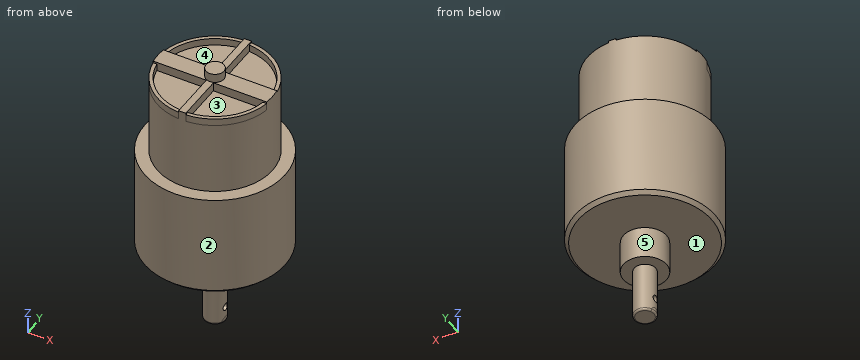
from build123d import *
from build123d.topology import SkipClean

# Parameters (mm, degrees)
SKETCH1_R               = 16
BOSS_EXTRUDE1_DEPTH     = 23
SKETCH2_R               = 19.5
BOSS_EXTRUDE2_DEPTH     = 29
SKETCH3_R               = 6
BOSS_EXTRUDE4_DEPTH     = 9
SKETCH4_R               = 3
BOSS_EXTRUDE5_DEPTH     = 22
CUT_EXTRUDE2_DEPTH      = 22
CUT_EXTRUDE2_DEPTH_BACK = 22
SKETCH5_R               = 1.5
CUT_EXTRUDE4_START      = -2.5
CUT_EXTRUDE4_DEPTH      = 2.5
SKETCH7_R               = 2.5
BOSS_EXTRUDE6_DEPTH     = 2.5
BOSS_EXTRUDE7_DEPTH     = 2
CHAMFER1_SIZE           = 1
FILLET1_R               = 1
BOSS_EXTRUDE8_START     = -22
SKETCH9_R               = 3
BOSS_EXTRUDE8_DEPTH     = 22
CUT_EXTRUDE6_START      = -8
SKETCH10_R              = 3
CUT_EXTRUDE6_DEPTH      = 8
FILLET2_R               = 0.5
CUT_EXTRUDE7_DEPTH      = 59.860003398
CUT_EXTRUDE7_DEPTH_BACK = 59.860003398
SKETCH11_R              = 1


with BuildPart() as part:
    # Sketch1 → Boss-Extrude1 (new body)
    with BuildSketch(Plane.XY):
        Circle(SKETCH1_R)
    extrude(amount=BOSS_EXTRUDE1_DEPTH)

    # Sketch2 → Boss-Extrude2 (add)
    with BuildSketch(Plane(origin=(0, 0, 0), x_dir=(-1, 0, 0), z_dir=(0, 0, -1))):
        with Locations(Location((0, 0, 0), (0, 0, 180))):
            Circle(SKETCH2_R)
    extrude(amount=BOSS_EXTRUDE2_DEPTH)

    # Sketch3 → Boss-Extrude4 (add)
    with BuildSketch(Plane(origin=(0, 0, -29), x_dir=(-1, 0, 0), z_dir=(0, 0, -1))):
        Circle(SKETCH3_R)
    extrude(amount=BOSS_EXTRUDE4_DEPTH)

    # Sketch4 → Boss-Extrude5 (add)
    with BuildSketch(Plane(origin=(0, 0, -38), x_dir=(-1, 0, 0), z_dir=(0, 0, -1))):
        Circle(SKETCH4_R)
    extrude(amount=BOSS_EXTRUDE5_DEPTH)

    # Sketch5 → Cut-Extrude2 (cut, two sides: drawn at the far end of the back side and taken through both)
    with BuildSketch(Plane(origin=(0, 0, 0), x_dir=(0, 0, -1), z_dir=(1, 0, 0)).offset(-CUT_EXTRUDE2_DEPTH_BACK)):
        with Locations((52, 0)):
            Circle(SKETCH5_R)
    extrude(amount=CUT_EXTRUDE2_DEPTH + CUT_EXTRUDE2_DEPTH_BACK, mode=Mode.SUBTRACT)

    # Sketch6 → Cut-Extrude4 (cut)
    with BuildSketch(Plane.XY.offset(23).offset(CUT_EXTRUDE4_START)):
        with BuildLine():
            Line((0.998052578, -2.481549033), (0.998052578, -15.968841256))
            ThreePointArc((0.998052578, -15.968841256), (10.773767775, -11.829029036), (15.806388405, -2.481549033))
            Line((15.806388405, -2.481549033), (0.998052578, -2.481549033))
        make_face()
        with BuildLine():
            Line((-0.998052578, 15.968841256), (-0.998052578, 2.481549033))
            Line((-0.998052578, 2.481549033), (-15.806388405, 2.481549033))
            ThreePointArc((-15.806388405, 2.481549033), (-10.773767775, 11.829029036), (-0.998052578, 15.968841256))
        make_face()
        with BuildLine():
            Line((0.998052578, 15.968841256), (0.998052578, 2.481549033))
            Line((0.998052578, 2.481549033), (15.806388405, 2.481549033))
            ThreePointArc((15.806388405, 2.481549033), (10.773767775, 11.829029036), (0.998052578, 15.968841256))
        make_face()
        with BuildLine():
            Line((-15.806388405, -2.481549033), (-0.998052578, -2.481549033))
            Line((-0.998052578, -2.481549033), (-0.998052578, -15.968841256))
            ThreePointArc((-0.998052578, -15.968841256), (-10.773767775, -11.829029036), (-15.806388405, -2.481549033))
        make_face()
    extrude(amount=CUT_EXTRUDE4_DEPTH, mode=Mode.SUBTRACT)

    # Sketch7 → Boss-Extrude6 (add)
    with BuildSketch(Plane.XY.offset(23)):
        Circle(SKETCH7_R)
    extrude(amount=BOSS_EXTRUDE6_DEPTH)

    # Sketch8 → Boss-Extrude7 (add)
    with BuildSketch(Plane.XY.offset(20.5)):
        with BuildLine():
            Line((-15.806388405, 2.481549033), (-14.793306405, 2.481549033))
            ThreePointArc((-14.793306405, 2.481549033), (-10.065380021, 11.12151631), (-0.998052578, 14.966759537))
            Line((-0.998052578, 14.966759537), (-0.998052578, 15.968841256))
            ThreePointArc((-0.998052578, 15.968841256), (-10.773767775, 11.829029036), (-15.806388405, 2.481549033))
        make_face()
        with BuildLine():
            Line((0.998052578, 15.968841256), (0.998052578, 14.966759537))
            ThreePointArc((0.998052578, 14.966759537), (10.065380021, 11.12151631), (14.793306405, 2.481549033))
            Line((14.793306405, 2.481549033), (15.806388405, 2.481549033))
            ThreePointArc((15.806388405, 2.481549033), (10.773767775, 11.829029036), (0.998052578, 15.968841256))
        make_face()
        with BuildLine():
            Line((15.806388405, -2.481549033), (14.793306405, -2.481549033))
            ThreePointArc((14.793306405, -2.481549033), (10.065380021, -11.12151631), (0.998052578, -14.966759537))
            Line((0.998052578, -14.966759537), (0.998052578, -15.968841256))
            ThreePointArc((0.998052578, -15.968841256), (10.773767775, -11.829029036), (15.806388405, -2.481549033))
        make_face()
        with BuildLine():
            Line((-0.998052578, -15.968841256), (-0.998052578, -14.966759537))
            ThreePointArc((-0.998052578, -14.966759537), (-10.065380021, -11.12151631), (-14.793306405, -2.481549033))
            Line((-14.793306405, -2.481549033), (-15.806388405, -2.481549033))
            ThreePointArc((-15.806388405, -2.481549033), (-10.773767775, -11.829029036), (-0.998052578, -15.968841256))
        make_face()
    extrude(amount=BOSS_EXTRUDE7_DEPTH)

    # Chamfer1
    chamfer1_edges = [part.edges().sort_by_distance(p)[0] for p in [
        (-19.5, 0, -29),
    ]]
    chamfer(chamfer1_edges, length=CHAMFER1_SIZE)

    # Fillet1
    fillet1_edges = [part.edges().sort_by_distance(p)[0] for p in [
        (3, 0, -60),
    ]]
    fillet(fillet1_edges, radius=FILLET1_R)

    # Sketch9 → Boss-Extrude8 (add)
    with SkipClean():  # the faces are left unmerged after this step: merging them gives an invalid solid
        with BuildSketch(Plane(origin=(0, 0, -60), x_dir=(-1, 0, 0), z_dir=(0, 0, -1)).offset(BOSS_EXTRUDE8_START)):
            Circle(SKETCH9_R)
        extrude(amount=BOSS_EXTRUDE8_DEPTH)

    # Sketch10 → Cut-Extrude6 (cut)
    with BuildSketch(Plane(origin=(0, 0, -60), x_dir=(-1, 0, 0), z_dir=(0, 0, -1)).offset(CUT_EXTRUDE6_START)):
        Circle(SKETCH10_R)
    extrude(amount=CUT_EXTRUDE6_DEPTH, mode=Mode.SUBTRACT)

    # Fillet2
    fillet2_edges = [part.edges().sort_by_distance(p)[0] for p in [
        (3, 0, -52),
    ]]
    fillet(fillet2_edges, radius=FILLET2_R)

    # Sketch11 → Cut-Extrude7 (cut, two sides: drawn at the far end of the back side and taken through both)
    with BuildSketch(Plane(origin=(0, 0, 0), x_dir=(0, 0, -1), z_dir=(1, 0, 0)).offset(-CUT_EXTRUDE7_DEPTH_BACK)):
        with Locations((47.584115537, 0)):
            Circle(SKETCH11_R)
    extrude(amount=CUT_EXTRUDE7_DEPTH + CUT_EXTRUDE7_DEPTH_BACK, mode=Mode.SUBTRACT)


solid = part.part
Geometry check sheet. Reference: the model listing, model coordinates, mm. Face numbers are marked on the shaded views. A direction names the side the tool comes from. Give positions to 0.01 mm unless a question says otherwise; leave off trailing zeros. Loops run counter-clockwise (first coordinate to the right, second up) from the corner with the lowest first, then second, coordinate; pieces in that order, holes last. Notation, with made-up numbers: M -22,19.5 L 21,19.5 A20 cw 21,39.5 Z; hole C 59,51.25 d8. An arc over 180 degrees is marked long. Answer as a JSON object with one key per item and string values. Group by question number.
Item 1: Access from +Z, -Z, +X, -X, +Y, -Y to the whole of each face (thin tool, end or side, straight path). Record for the marked faces 4 and 5.
Item 2: Material ranges on L1, parallel to Y at x = -2.5, z = 21.5; L2, parallel to Z at x = 0.75, y = 0; L3, parallel to Y at x = -9, z = 22, recorded low to high.
Item 3: Sectioned sample at A-A on y = 0. Record the boundary of the cut face in (x, z).
Item 4: Sectioned sample at B-B on x = 0. Record the boundary of the cut face in (y, z).
Item 5: Sectioned sample at C-C on z = -19. Record the boundary of the cut face in (x, y).
Item 6: Gauge pin test, flat ends, axial feed: pin 1 (1.5 mm diameter, centred on x = -5.5, y = 6.5, fed in from +Z); pin 2 (1.2 mm diameter, centred on x = -5, z = 22, fed in from +Y); pin 3 (4 mm diameter, centred on y = -10.5, z = -31.5, fed in from -X); pin 4 (6 mm diameter, centred on y = 6, z = -2, fed in from +X). Record the tip position at first contact, or that the pin passes through.
Item 7: Mould release check, pull along X, two halves, no side actions. Record for the marked faces 1, 2 and 3: pulls with the +X half, pulls with the -X half, needs draft (parallel to the pull), parting line crosses it, or undercut.
Findings below:
{
 "1": {"face 4": "+Z", "face 5": "-Z"},
 "2": {"L1": "-15.8 to -14.79, -2.48 to 2.48, 14.79 to 15.8", "L2": "-52 to -48.58, -46.58 to 25.5", "L3": "-13.23 to -12, -2.48 to 2.48, 12 to 13.23"},
 "3": {"outline": "M -19.5,-28 L -18.5,-29 L -6,-29 L -6,-38 L -3,-38 L -3,-46.58 L 3,-46.58 L 3,-38 L 6,-38 L 6,-29 L 18.5,-29 L 19.5,-28 L 19.5,0 L 16,0 L 16,23 L 2.5,23 L 2.5,25.5 L -2.5,25.5 L -2.5,23 L -16,23 L -16,0 L -19.5,0 Z; M -3,-51.5 A0.5 ccw -2.5,-52 L 2.5,-52 A0.5 ccw 3,-51.5 L 3,-48.58 L -3,-48.58 Z"},
 "4": {"outline": "M -19.5,-28 L -18.5,-29 L -6,-29 L -6,-38 L -3,-38 L -3,-51.5 A0.5 ccw -2.5,-52 L 2.5,-52 A0.5 ccw 3,-51.5 L 3,-38 L 6,-38 L 6,-29 L 18.5,-29 L 19.5,-28 L 19.5,0 L 16,0 L 16,23 L 2.5,23 L 2.5,25.5 L -2.5,25.5 L -2.5,23 L -16,23 L -16,0 L -19.5,0 Z; hole C 0,-47.58 d2"},
 "5": {"outline": "C 0,0 d39"},
 "6": {"pin 1": "z = 20.5", "pin 2": "y = 15.38", "pin 3": "through", "pin 4": "x = 19.27"},
 "7": {"face 1": "needs draft", "face 2": "parting line crosses it", "face 3": "undercut"}
}
